Job drawing, mm, ordinate dimensions from the low corner. One solid piece. Coordinates: 2 decimals unless noted, no trailing zeros. Order: outer loops, then holes, each group sorted by start corner. A loop starts at its lowest first (then second) coordinate and runs counter-clockwise, first axis right, second up. Notation, with made-up numbers: (36.5, 28.5) -> (81.5, 28.5) arc R16 cw to (81.5, 40.5) -> close; hole circle Ø6 at (41.5, 65). An arc over 180 degrees is marked (long way). Use CSV: the item, a comma, the result in double quotes. Start each with the question number.
(1) Cut at A-A on x = 11. Write the cut outline in (y, z).
(2) Probe L1, parallel to Z at x = 47, y = 2.2; L2, parallel to Z at x = 46, y = 2.2; L3, parallel to X at y = 0.25, z = 47.5. List the from-to ranges inside material, lowest first.
(3) Cut at B-B on z = 48. Write the cut outline in (x, y).
(4) Pin check, flat tips, straight feed: pin 1 Ø0.9 at (x, y) = (2, 1) entering from +Z; pin 2 Ø0.9 at (y, z) = (1.5, 88.5) entering from +X; pin 3 Ø0.9 at (y, z) = (2, 24.5) entering from +X. Stop position of each tip, or through.
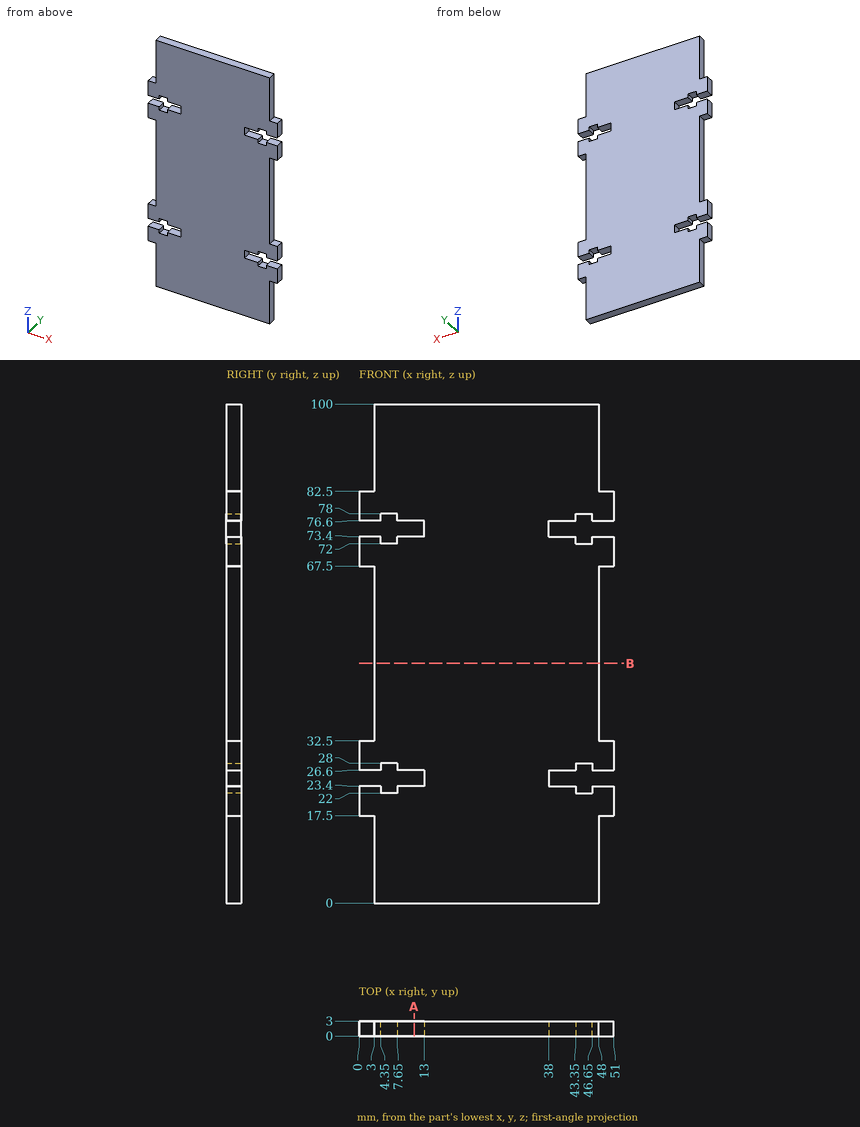
Outcome:
1,outline,"(0, 0) -> (3, 0) -> (3, 23.4) -> (0, 23.4) -> close; (0, 26.6) -> (3, 26.6) -> (3, 73.4) -> (0, 73.4) -> close; (0, 76.6) -> (3, 76.6) -> (3, 100) -> (0, 100) -> close"
2,L1,"0 to 23.4, 26.6 to 73.4, 76.6 to 100"
2,L2,"0 to 22, 28 to 72, 78 to 100"
2,L3,"3 to 48"
3,outline,"(3, 0) -> (48, 0) -> (48, 3) -> (3, 3) -> close"
4,pin 1,"z = 82.5"
4,pin 2,"x = 48"
4,pin 3,"x = 38"
